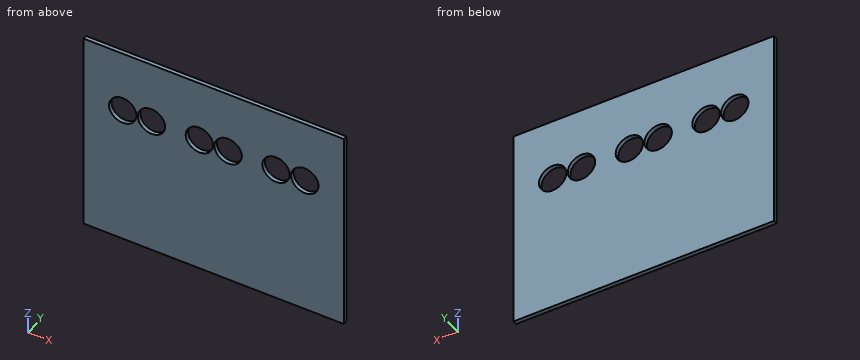
```python
from build123d import *

# Parameters (mm, degrees)
SKETCH1_W          = 190
SKETCH1_H          = 150
SKETCH1_R          = 10
BASE_FLANGE1_DEPTH = 3


# Sheet-metal steps are written as plain solids
with BuildPart() as part:
    # Sketch1 → Base-Flange1 (new body)
    with BuildSketch(Plane(origin=(0, 0, 0), x_dir=(1, 0, 0), z_dir=(0, 1, 0))):
        with Locations((95, 75)):
            Rectangle(SKETCH1_W, SKETCH1_H)
        with Locations(Location((28.5, 46, 0), (0, 0, 270))):
            Circle(SKETCH1_R, mode=Mode.SUBTRACT)
        with Locations(Location((49.5, 46, 0), (0, 0, 270))):
            Circle(SKETCH1_R, mode=Mode.SUBTRACT)
        with Locations(Location((84.5, 46, 0), (0, 0, 270))):
            Circle(SKETCH1_R, mode=Mode.SUBTRACT)
        with Locations(Location((105.5, 46, 0), (0, 0, 270))):
            Circle(SKETCH1_R, mode=Mode.SUBTRACT)
        with Locations(Location((140.5, 46, 0), (0, 0, 270))):
            Circle(SKETCH1_R, mode=Mode.SUBTRACT)
        with Locations(Location((161.5, 46, 0), (0, 0, 270))):
            Circle(SKETCH1_R, mode=Mode.SUBTRACT)
    extrude(amount=-BASE_FLANGE1_DEPTH)


solid = part.part
```
Check sheet for the modelled part. Datum: model origin and axes. Units: mm. Round coordinates to 2 decimals unless told otherwise and drop trailing zeros. Order: outer loops, then holes, each group sorted by start corner. A loop starts at its lowest first (then second) coordinate and runs counter-clockwise, first axis right, second up. Notation, with made-up numbers: (64.25, 26.5) -> (99.25, 26.5) arc R16 cw to (99.25, 44.5) -> close; hole circle Ø3 at (77, 23). An arc over 180 degrees is marked (long way). One line per item, written item: value. Start each with the question number.
Q1. Cross-section at B-B (y = -2.3). Record the boundary of the cut face in (x, z).
Q2. Thickness scan on line 1 (Z direction, x = 32.5, y = -0.75); line 2 (Z direction, x = 57, y = -0.55). Record the ranges inside material, lowest first.
Q3. Cross-section at A-A (x = 49.5). Record the boundary of the cut face in (y, z).
Q4. Cross-section at C-C (x = 26.5). Record the boundary of the cut face in (y, z), and give its area (3 significant figures).
Completed:
1. outline: (0, -150) -> (190, -150) -> (190, 0) -> (0, 0) -> close; hole circle Ø20 at (28.5, -46); hole circle Ø20 at (49.5, -46); hole circle Ø20 at (84.5, -46); hole circle Ø20 at (105.5, -46); hole circle Ø20 at (140.5, -46); hole circle Ø20 at (161.5, -46)
2. line 1: z = -150 to -55.17, -36.83 to 0
2. line 2: z = -150 to -52.61, -39.39 to 0
3. outline: (-3, -150) -> (0, -150) -> (0, -56) -> (-3, -56) -> close; (-3, -36) -> (0, -36) -> (0, 0) -> (-3, 0) -> close
4. outline: (-3, -150) -> (0, -150) -> (0, -55.8) -> (-3, -55.8) -> close; (-3, -36.2) -> (0, -36.2) -> (0, 0) -> (-3, 0) -> close
4. area: 391 mm²
